Can you work these out from the model? Positions are in its coordinate system, mm. Round coordinates to 2 decimals unless told otherwise and drop trailing zeros. Order: outer loops, then holes, each group sorted by start corner. A loop starts at its lowest first (then second) coordinate and runs counter-clockwise, first axis right, second up.
Autodesk Inventor part; units mm, degrees
ref_plane "YZ Plane" through (0, 0, 0) normal (1, 0, 0) x (0, 1, 0)
ref_plane "XZ Plane" through (0, 0, 0) normal (0, 1, 0) x (-1, 0, 0)
ref_plane "XY Plane" through (0, 0, 0) normal (0, 0, 1) x (1, 0, 0)
sketch "スケッチ1" plane through (0, 0, 0) normal (0, 0, 1) x (1, 0, 0)
  circle A0 centre (0, 0) radius 1.5
  dimension "d0" = 3
extrude "押し出し1" add sketch "スケッチ1" along normal blind 6
sketch "スケッチ2" plane through (0, 0, 6) normal (0, 0, 1) x (1, 0, 0)
  circle A0 centre (0, 0) radius 1.5
  circle A1 centre (0, 0) radius 3
  dimension "d3" = 6
extrude "押し出し2" add sketch "スケッチ2" along normal blind 1.75 contours A0 | A1
thread "ねじ1"
chamfer "面取り1" distance 1.5 angle 45 1 edges at (-3, 0, 6)
sketch "スケッチ4" plane through (0, 0, 0) normal (0, 0, -1) x (-1, 0, 0)
  circle A0 centre (0, 0) radius 1.5
extrude "押し出し4" add sketch "スケッチ4" along normal blind 4
sketch "スケッチ5" plane through (0, 0, -4) normal (0, 0, -1) x (-1, 0, 0)
  circle A0 centre (0, 0) radius 1.5
extrude "押し出し5" cut sketch "スケッチ5" against normal blind 2
sketch "スケッチ6" plane through (0, 0, -2) normal (0, 0, -1) x (-1, 0, 0)
  circle A0 centre (0, 0) radius 1.5
extrude "押し出し6" add sketch "スケッチ6" along normal blind 6.25
properties part number "SB　16mm皿ネジ" material "Steel, Mild"
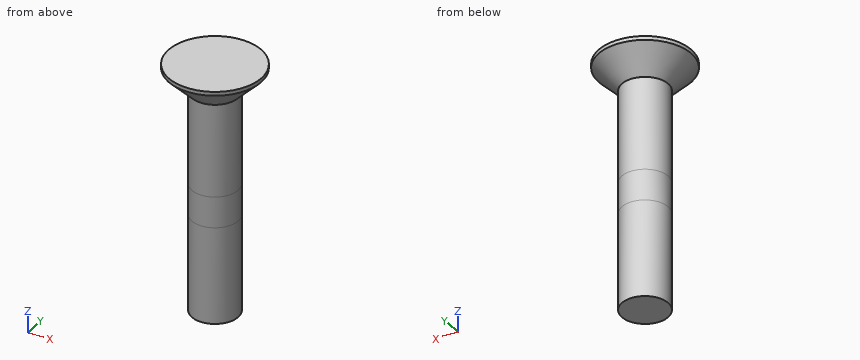
(1) Please list where these lines run through material, in increasing order: probe 1 along X at (y, z) = (-0.05, 4.75); probe 2 along Z at (x, y) = (-1.9, 1).
(2) I want a section at C-C, the plane z = -0.25. List the corners of the cut face in (x, y) for me.
(3) I'm going to push a flat-ended pin straight in: pin 1 Ø2 at (y, z) = (0.5, 2) entering from -X. Where does the tip first touch, or does it pass through?
Ans:
1. probe 1: x = -1.5 to 1.5
1. probe 2: z = 6.65 to 7.75
2. outline: circle Ø3 at (0, 0)
3. pin 1: stops at x = -1.5
